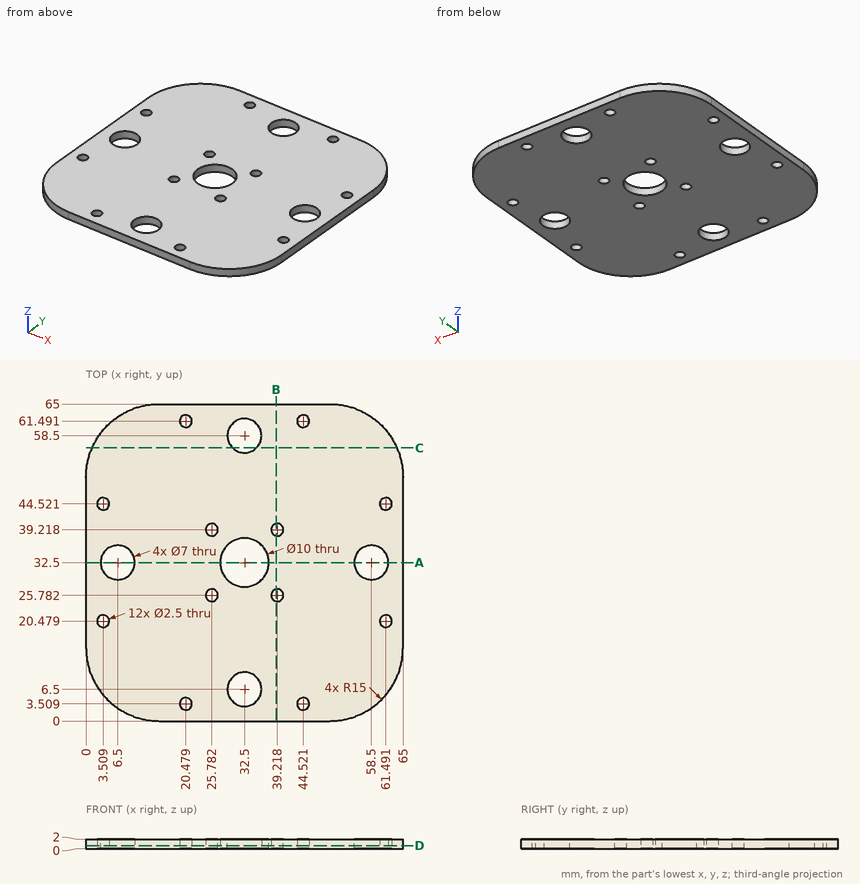
Part print with two shaded views. Sizes in mm from the minimum x, y, z corner. Round coordinates to 2 decimals unless told otherwise and drop trailing zeros. Loops run counter-clockwise (first coordinate to the right, second up) from the corner with the lowest first, then second, coordinate; pieces in that order, holes last.
Item 1: Drill centre lines: line 1 along Y through (x, z) = (38.5, 0.5) (1 decimal); line 2 along X through (y, z) = (60.5, 0.95) (1 decimal); line 3 along Y through (x, z) = (32.5, 1). Where is each one in solid material? Low to high.
Item 2: Saw through at D-D (z = 0.65). State how many separate pieces and enclosed holes the cut face has, then the cut area to 3 significant figures.
Item 3: Saw through at A-A (y = 32.5). List the corners of the cut face in (x, z).
Item 4: Saw through at B-B (x = 39). List the corners of the cut face in (y, z).
Item 5: Pin check, flat tip, straight feed: P1, Ø2, axis at x = 61.49, y = 44.52, coming from the +Z side. Stop position of the tip, or through.
Item 6: Saw through at C-C (y = 56). List the corners of the cut face in (x, z), then the cut area to 3 significant figures.
Worked answers:
1. line 1: y = 0 to 24.8, 26.8 to 38.2, 40.2 to 65
1. line 2: x = 4.3 to 19.7, 21.2 to 29.6, 35.4 to 43.8, 45.3 to 60.7
1. line 3: y = 0 to 3, 10 to 27.5, 37.5 to 55, 62 to 65
2. separate pieces: 1
2. enclosed holes: 17
2. area: 3,740 mm2
3. outline: (0, 0) - (3, 0) - (3, 2) - (0, 2) - close; (10, 0) - (27.5, 0) - (27.5, 2) - (10, 2) - close; (37.5, 0) - (55, 0) - (55, 2) - (37.5, 2) - close; (62, 0) - (65, 0) - (65, 2) - (62, 2) - close
4. outline: (0, 0) - (24.55, 0) - (24.55, 2) - (0, 2) - close; (27.01, 0) - (37.99, 0) - (37.99, 2) - (27.01, 2) - close; (40.45, 0) - (65, 0) - (65, 2) - (40.45, 2) - close
5. P1: passes through
6. outline: (1.25, 0) - (30.05, 0) - (30.05, 2) - (1.25, 2) - close; (34.95, 0) - (63.75, 0) - (63.75, 2) - (34.95, 2) - close
6. area: 115 mm2
